Geometry check sheet. Reference: drawing and pictorial views, mm from the part's lowest x, y, z. Give positions to 0.01 mm unless a question says otherwise; leave off trailing zeros. Write each loop counter-clockwise with the first axis right and the second up, starting at its lowest first coordinate (ties: lowest second). Pieces come first, ordered by that corner, then holes.
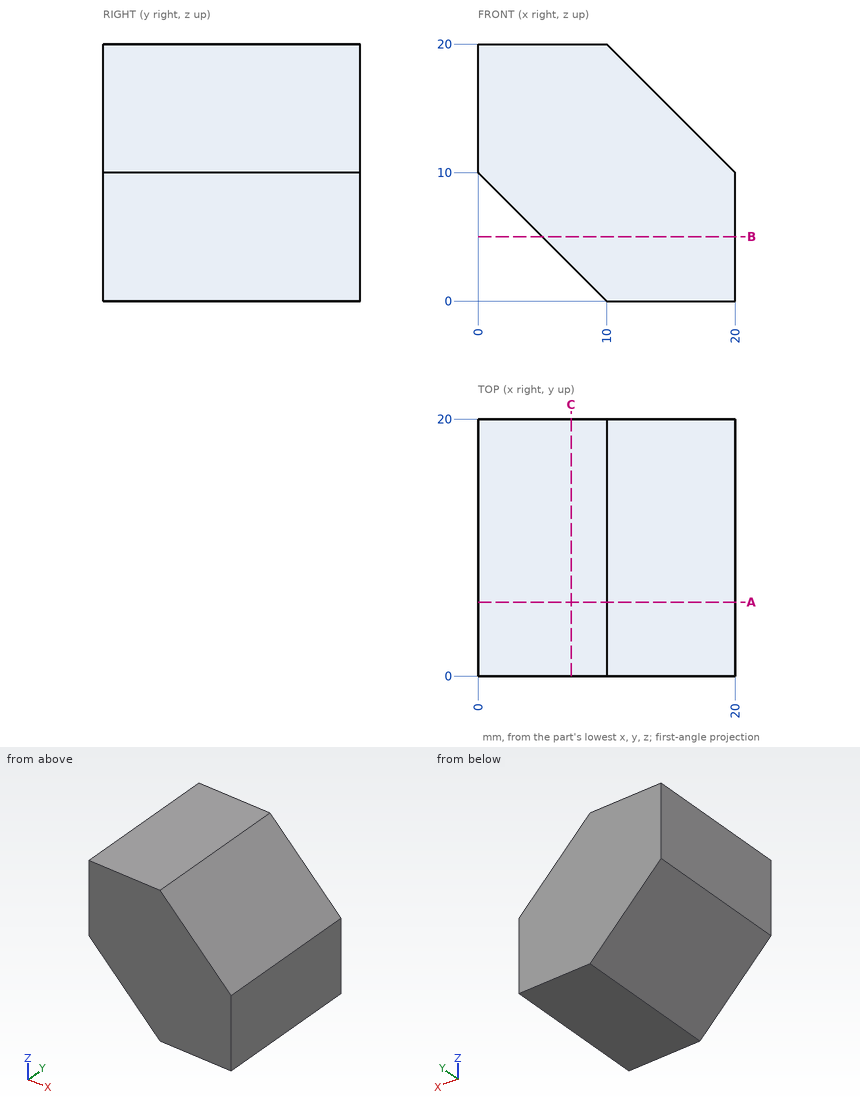
Item 1: Sectioned sample at C-C on x = 7.25. Record the cut outline in (y, z).
Answer key:
outline: (0, 2.75) - (20, 2.75) - (20, 20) - (0, 20) - close
Item 2: Sectioned sample at A-A on y = 5.75. Record the cut outline in (x, z).
Answer key:
outline: (0, 10) - (10, 0) - (20, 0) - (20, 10) - (10, 20) - (0, 20) - close
Item 3: Depth check by flat-ended pin: pin 1 (2 mm diameter, centred on y = 15.5, z = 11.5, fed in from +X); pin 2 (5 mm diameter, centred on x = 13, z = 14.5, fed in from -Y); pin 3 (8 mm diameter, centred on y = 10.5, z = 3, fed in from -X). Enter the tip coordinate at first touch or a pass-through.
Answer key:
pin 1: stops at x = 19.5
pin 2: stops at y = 0
pin 3: stops at x = 3
Item 4: Sectioned sample at B-B on z = 5. Record the cut outline in (x, y), then the cut area to 3 significant figures.
Answer key:
outline: (5, 0) - (20, 0) - (20, 20) - (5, 20) - close
area: 300 mm2
Item 5: Scan lines: line 1 along Z through (x, y) = (3.75, 2); line 2 along X through (y, z) = (5.5, 10.5); line 3 along Z through (x, y) = (12.5, 16.75). Record each from-to range of solid material in increasing order.
Answer key:
line 1: z = 6.25 to 20
line 2: x = 0 to 19.5
line 3: z = 0 to 17.5
